Autodesk Inventor part; units mm, degrees
ref_plane "YZ Plane" through (0, 0, 0) normal (1, 0, 0) x (0, 1, 0)
ref_plane "XZ Plane" through (0, 0, 0) normal (0, 1, 0) x (-1, 0, 0)
ref_plane "XY Plane" through (0, 0, 0) normal (0, 0, 1) x (1, 0, 0)
sketch "Szkic1" plane through (0, 0, 0) normal (0, 1, 0) x (-1, 0, 0)
  line L0 (34.6, 10.4209) -> (34.6, 8.4209)
  line L1 (34.6, 8.4209) -> (50, 8.4209)
  line L2 (50, 8.4209) -> (50, 10.4209)
  line L3 (50, 10.4209) -> (34.6, 10.4209)
  line L4 (0, 0) -> (0, 76.2035)
  dimension "d0" = 15.4
  dimension "d1" = 2
  dimension "d2" = 34.6
revolve "Obrót1" add sketch "Szkic1" angle 360 about axis through (0, 0, 0) along (0, 0, 1)
sketch "Szkic2" plane through (0, 0, 10.4209) normal (0, 0, 1) x (1, 0, 0)
  circle A0 centre (0, 0) radius 40.3
  circle A1 centre (0, 40.3) radius 3.05
  dimension "d4" = 80.6
  dimension "d5" = 6.1
extrude "Wyciągnięcie proste1" cut sketch "Szkic2" against normal blind 10 contours A1 A0 | A0 A1 picked at (-0.1196, 39.2818) picked at (0.1049, 41.3027)
sketch "Szkic3" plane through (0, 0, 10.4209) normal (0, 0, 1) x (1, 0, 0)
  circle A0 centre (0, 0) radius 40.3
  circle A1 centre (40.3, 0) radius 3.05
  circle A2 centre (0, -40.3) radius 3.05
  circle A3 centre (-40.3, 0) radius 3.05
  dimension "d8" = 80.6
  dimension "d9" = 6.1
  dimension "d10" = 6.1
  dimension "d11" = 6.1
extrude "Wyciągnięcie proste2" cut sketch "Szkic3" against normal blind 10 contours A0 A1 | A0 A1 | A3 A0 | A0 A3 | A2 A0 | A0 A2
properties part number "uszczelka" material "Poliwęglan dymiony"
Read the model definition and answer for the solid it produces. Units are mm, in the model's axes. Coordinates: 2 decimals unless noted, no trailing zeros. Write each loop counter-clockwise with the first axis right and the second up, starting at its lowest first coordinate (ties: lowest second). Pieces come first, ordered by that corner, then holes. Notation, with made-up numbers: (67.25, 25) -> (77.25, 25) arc R30 cw to (77.25, 53) -> close; hole circle Ø9 at (76, 39.5). An arc over 180 degrees is marked (long way). Return JSON: item names as keys, results as strings.
(1) The part is cut by section B-B on x = -11.5. Give the vertices of the cut face in (y, z).
Answers below:
{"outline": "(-48.66, 8.42) -> (-32.63, 8.42) -> (-32.63, 10.42) -> (-48.66, 10.42) -> close; (32.63, 8.42) -> (48.66, 8.42) -> (48.66, 10.42) -> (32.63, 10.42) -> close"}
(2) The part is cut by section C-C on z = 10.1. Give the vertices of the cut face in (x, y), then the cut area to 3 significant figures.
Answers below:
{"outline": "circle Ø100 at (0, 0); hole circle Ø6.1 at (-40.3, 0); hole circle Ø69.2 at (0, 0); hole circle Ø6.1 at (0, -40.3); hole circle Ø6.1 at (0, 40.3); hole circle Ø6.1 at (40.3, 0)", "area": "3,980 mm^2"}
(3) The part is cut by section D-D on y = 40.3. Give the vertices of the cut face in (x, z).
Answers below:
{"outline": "(-29.6, 8.42) -> (-3.05, 8.42) -> (-3.05, 10.42) -> (-29.6, 10.42) -> close; (3.05, 8.42) -> (29.6, 8.42) -> (29.6, 10.42) -> (3.05, 10.42) -> close"}
(4) This flat-tipped pin is pushed along its axis until it touches: P1, Ø10, axis at x = 40.3, y = 0, coming from the -Z side. Where does it stop, or does it pass through?
Answers below:
{"P1": "z = 8.42"}
(5) For a pull along X with two mould halves and no side action, classify faces 1 (the cylindrical face through (-33, 10.4, 9.4)), 2 (the cylindrical face through (-47.69, -15.02, 9.43)), 3 (the flat face through (12, 33, 8.421)) as pulls with the +X half, pulls with the -X half, needs draft (parallel to the pull), parting line crosses it, or undercut.
Answers below:
{"face 1": "undercut", "face 2": "parting line crosses it", "face 3": "needs draft"}
(6) Consider line 1 along X through (y, z) = (0, 9); line 2 along Y through (x, z) = (24, 9.5). Determine where each line is inside the solid, lowest interval first. Write a range as from..to.
Answers below:
{"line 1": "-50..-43.35, -37.25..-34.6, 34.6..37.25, 43.35..50", "line 2": "-43.86..-24.92, 24.92..43.86"}
(7) The part is cut by section A-A on y = 0. Give the vertices of the cut face in (x, z), then the cut area to 3 significant figures.
Answers below:
{"outline": "(-50, 8.42) -> (-43.35, 8.42) -> (-43.35, 10.42) -> (-50, 10.42) -> close; (-37.25, 8.42) -> (-34.6, 8.42) -> (-34.6, 10.42) -> (-37.25, 10.42) -> close; (34.6, 8.42) -> (37.25, 8.42) -> (37.25, 10.42) -> (34.6, 10.42) -> close; (43.35, 8.42) -> (50, 8.42) -> (50, 10.42) -> (43.35, 10.42) -> close", "area": "37.2 mm^2"}
